```python
from build123d import *

# Parameters (mm, degrees)
F0_R     = 15
F1_DEPTH = 75
F3_DEPTH = 10


with BuildPart() as f1:
    # F0 (on Front) → F1 (new body, symmetric)
    with BuildSketch(Plane.XZ):
        Circle(F0_R)
    extrude(amount=F1_DEPTH, both=True)

    # F2 (on face) → F3 (join)
    with BuildSketch(Plane.XZ.offset(75)):
        Polygon((28.369565, 0), (14.184782, 24.568764), (-14.184782, 24.568764), (-28.369565, 0), (-14.184782, -24.568764), (14.184782, -24.568764), align=None)
    extrude(amount=F3_DEPTH)


solid = f1.part
```
Could you check a few things on this model? Use its own coordinates, in mm. A direction names the side the tool comes from. Coordinates: 2 decimals unless noted, no trailing zeros. Write each loop counter-clockwise with the first axis right and the second up, starting at its lowest first coordinate (ties: lowest second). Pieces come first, ordered by that corner, then holes. Notation, with made-up numbers: (47.5, 2) -> (84.5, 2) arc R29 ccw to (84.5, 25) -> close; hole circle Ø5 at (22.5, 81). An arc over 180 degrees is marked (long way). One line per question, with ' | ' between items. Start each with the question number.
1. If we section it at C-C (y = 61): Please give me the cut outline in (x, z), and give its area (3 significant figures).
2. If we section it at A-A (x = 9): Please give me the cut outline in (y, z), and give its area (3 significant figures).
3. If we section it at B-B (z = -5.5): Please give me the cut outline in (x, y).
4. Will these pins go through, and if not, where does the flat tip stop? P1, Ø12, axis at x = 14, y = 21, coming from the +Z side; P2, Ø3, axis at x = 12, y = 41.5, coming from the -Z side; P3, Ø2, axis at y = -14.5, z = 13, coming from the +X side.
5. For faces 1 (the face through (12, -75, -11)), 2 (the face through (0, -80, 24.569)), which set-ups out of +Z, -Z, +X, -X, +Y, -Y let a thin tool reach every point of the face, with its end or its side?
6. Please list where these lines run through material, in increasing order: line 1 along Y through (x, z) = (12, -21.5); line 2 along Z through (x, y) = (0.5, 37); line 3 along Z through (x, y) = (3.5, 4).
7. If we section it at D-D (x = -23.5): Please give me the cut outline in (y, z).
Return value:
1) outline: circle Ø30 at (0, 0) | area: 707 mm²
2) outline: (-85, -24.57) -> (-75, -24.57) -> (-75, -12) -> (75, -12) -> (75, 12) -> (-75, 12) -> (-75, 24.57) -> (-85, 24.57) -> close | area: 4,090 mm²
3) outline: (-25.19, -85) -> (25.19, -85) -> (25.19, -75) -> (13.96, -75) -> (13.96, 75) -> (-13.96, 75) -> (-13.96, -75) -> (-25.19, -75) -> close
4) P1: stops at z = 12.69 | P2: stops at z = -10.71 | P3: stops at x = 9
5) face 1: +Y | face 2: +Z, +X, -X, +Y, -Y
6) line 1: y = -85 to -75 | line 2: z = -14.99 to 14.99 | line 3: z = -14.59 to 14.59
7) outline: (-85, -8.43) -> (-75, -8.43) -> (-75, 8.43) -> (-85, 8.43) -> close
